from build123d import *

# Parameters (mm, degrees)
PAD_DEPTH                  = 2
PAD001_DEPTH               = 33
POCKET_DEPTH               = 133.8763
POCKET001_DEPTH            = 155.7439
PAD_MIRRORED_2_DEPTH       = 2
PAD001_MIRRORED_2_DEPTH    = 33
POCKET_MIRRORED_2_DEPTH    = 133.8763
POCKET001_MIRRORED_2_DEPTH = 155.7439


with BuildPart() as part:
    # Sketch → Pad (new body)
    with BuildSketch(Plane.XY):
        with BuildLine():
            ThreePointArc((5, 0), (3.535534, 3.535534), (0, 5))
            Line((0, 5), (0, 20))
            Line((0, 20), (39.191836, 20))
            ThreePointArc((41.867601, 13.531593), (40.658555, 16.819092), (39.191836, 20))
            Line((41.867601, 13.531593), (41.867601, 0))
            Line((41.867601, 0), (5, 0))
        make_face()
    pad = extrude(amount=PAD_DEPTH)

    # Sketch001 → Pad001 (join)
    with BuildSketch(Plane.XY):
        with BuildLine():
            ThreePointArc((41.867601, 13.531593), (40.658555, 16.819092), (39.191836, 20))
            Line((0, 20), (39.191836, 20))
            Line((0, 17.6), (0, 20))
            Line((37.030258, 17.6), (0, 17.6))
            ThreePointArc((39.467601, 11.104436), (38.386569, 14.403865), (37.030258, 17.6))
            Line((39.467601, 11.104436), (39.467601, 0))
            Line((39.467601, 0), (41.867601, 0))
            Line((41.867601, 0), (41.867601, 13.531593))
        make_face()
    pad001 = extrude(amount=PAD001_DEPTH)

    # Sketch002 → Pocket (cut, through all)
    with BuildSketch(Plane.XZ):
        Polygon((0, 10), (33.030258, 10), (33.030258, 19), (37.030258, 23), (37.030258, 33), (0, 33), align=None)
    pocket = extrude(amount=-POCKET_DEPTH, mode=Mode.SUBTRACT)

    # Sketch003 → Pocket001 (cut, through all)
    with BuildSketch(Plane.YZ):
        with BuildLine():
            Line((0, 15.000035), (0, 33))
            Line((0, 33), (13, 33))
            Line((13, 28), (13, 33))
            ThreePointArc((0, 15.000035), (9.192376, 18.807634), (13, 28))
        make_face()
    pocket001 = extrude(amount=POCKET001_DEPTH, mode=Mode.SUBTRACT)

    # Sketch Mirrored 2 → Pad Mirrored 2 (add)
    with BuildSketch(Plane(origin=(0, 0, 0), x_dir=(-1, 0, 0), z_dir=(0, 0, -1))):
        with BuildLine():
            ThreePointArc((5, 0), (3.535534, 3.535534), (0, 5))
            Line((0, 5), (0, 20))
            Line((0, 20), (39.191836, 20))
            ThreePointArc((41.867601, 13.531593), (40.658555, 16.819092), (39.191836, 20))
            Line((41.867601, 13.531593), (41.867601, 0))
            Line((41.867601, 0), (5, 0))
        make_face()
    pad_mirrored_2 = extrude(amount=-PAD_MIRRORED_2_DEPTH)

    # Sketch001 Mirrored 2 → Pad001 Mirrored 2 (add)
    with BuildSketch(Plane(origin=(0, 0, 0), x_dir=(-1, 0, 0), z_dir=(0, 0, -1))):
        with BuildLine():
            ThreePointArc((41.867601, 13.531593), (40.658555, 16.819092), (39.191836, 20))
            Line((0, 20), (39.191836, 20))
            Line((0, 17.6), (0, 20))
            Line((37.030258, 17.6), (0, 17.6))
            ThreePointArc((39.467601, 11.104436), (38.386569, 14.403865), (37.030258, 17.6))
            Line((39.467601, 11.104436), (39.467601, 0))
            Line((39.467601, 0), (41.867601, 0))
            Line((41.867601, 0), (41.867601, 13.531593))
        make_face()
    pad001_mirrored_2 = extrude(amount=-PAD001_MIRRORED_2_DEPTH)

    # Sketch002 Mirrored 2 → Pocket Mirrored 2 (cut, through all)
    with BuildSketch(Plane(origin=(0, 0, 0), x_dir=(-1, 0, 0), z_dir=(0, 1, 0))):
        Polygon((0, 10), (33.030258, 10), (33.030258, 19), (37.030258, 23), (37.030258, 33), (0, 33), align=None)
    pocket_mirrored_2 = extrude(amount=POCKET_MIRRORED_2_DEPTH, mode=Mode.SUBTRACT)

    # Sketch003 Mirrored 2 → Pocket001 Mirrored 2 (cut, through all)
    with BuildSketch(Plane.YZ):
        with BuildLine():
            Line((0, 15.000035), (0, 33))
            Line((0, 33), (13, 33))
            Line((13, 28), (13, 33))
            ThreePointArc((0, 15.000035), (9.192376, 18.807634), (13, 28))
        make_face()
    pocket001_mirrored_2 = extrude(amount=-POCKET001_MIRRORED_2_DEPTH, mode=Mode.SUBTRACT)

    # Mirrored001: Pad, Pad001, Pocket, Pocket001, Pad Mirrored 2, Pad001 Mirrored 2, Pocket Mirrored 2, Pocket001 Mirrored 2 across Sketch H_Axis
    add(pad.mirror(Plane.ZX))
    add(pad001.mirror(Plane.ZX))
    add(pocket.mirror(Plane.ZX), mode=Mode.SUBTRACT)
    add(pocket001.mirror(Plane.ZX), mode=Mode.SUBTRACT)
    add(pad_mirrored_2.mirror(Plane.ZX))
    add(pad001_mirrored_2.mirror(Plane.ZX))
    add(pocket_mirrored_2.mirror(Plane.ZX), mode=Mode.SUBTRACT)
    add(pocket001_mirrored_2.mirror(Plane.ZX), mode=Mode.SUBTRACT)


solid = part.part
The model under review builds one solid part; all positions refer to its coordinate system, in mm. A direction names the side the tool comes from. Coordinates: 2 decimals unless noted, no trailing zeros. Loops run counter-clockwise (first coordinate to the right, second up) from the corner with the lowest first, then second, coordinate; pieces in that order, holes last.
(1) Consider section A-A, the plane z = 7. Give the boundary of the cut face in (x, y), plus the area to 3 significant figures.
Determined:
outline: (-41.87, -13.53) arc R44 ccw to (-39.19, -20) - (39.19, -20) arc R44 ccw to (41.87, -13.53) - (41.87, 13.53) arc R44 ccw to (39.19, 20) - (-39.19, 20) arc R44 ccw to (-41.87, 13.53) - close; hole (-39.47, -11.1) arc R41 ccw to (-37.03, -17.6) - (37.03, -17.6) arc R41 ccw to (39.47, -11.1) - (39.47, 11.1) arc R41 ccw to (37.03, 17.6) - (-37.03, 17.6) arc R41 ccw to (-39.47, 11.1) - close
area: 568 mm2
(2) Draft analysis for pull direction Y (two halves, no side actions). For faces 6 (the flat face through (40, 13, 30)), 7 (the cylindrical face through (40.68, -16.77, 16.27)), 8 (the flat face through (39, -17, 33)), state which applies: +Y half, -Y half, draft (parallel to the pull), parting line (faces both ways), or undercut.
Determined:
face 6: undercut
face 7: -Y half
face 8: draft
(3) Wall thickness on L1, parallel to Y at x = 21, z = 3; L2, parallel to X at y = 8, z = 7; L3, parallel to X at y = -13, z = 10.5: over which ranges is each line inside the solid? List them lowest first.
Determined:
L1: y = -20 to -17.6, 17.6 to 20
L2: x = -41.87 to -39.47, 39.47 to 41.87
L3: x = -41.87 to -38.88, 38.88 to 41.87
(4) Insertion check: P1, Ø1.9, axis at y = -19, z = 15, coming from the -X side; P2, Ø0.7, axis at y = -18.5, z = 16, coming from the +X side; P3, Ø2.5, axis at x = 41, z = 30.5, coming from the -Y side. Each pin has a flat end and moves straight along its axis. Give the tip position at first contact, or say it passes through.
Determined:
P1: stops at x = -40.13
P2: stops at x = 40.08
P3: stops at y = -18.87
(5) Consider section D-D, the plane x = 13. Give the boundary of the cut face in (y, z), plus the area to 3 significant figures.
Determined:
outline: (-20, 0) - (20, 0) - (20, 10) - (17.6, 10) - (17.6, 2) - (-17.6, 2) - (-17.6, 10) - (-20, 10) - close
area: 118 mm2
(6) Consider section B-B, the plane y = -3.5. Give the boundary of the cut face in (x, z).
Determined:
outline: (-41.87, 0) - (-3.57, 0) - (-3.57, 2) - (-39.47, 2) - (-39.47, 15.48) - (-41.87, 15.48) - close; (3.57, 0) - (41.87, 0) - (41.87, 15.48) - (39.47, 15.48) - (39.47, 2) - (3.57, 2) - close
(7) Tool access review of faces 1 (the flat face through (0, -19, 10)), 2 (the flat face through (-39.468, 0, 9)), 3 (the flat face through (-39, -17, 33)), 4 (the flat face through (-1, -9, 0)), 5 (the flat face through (-40, 13, 30)): name each direction out of +Z, -Z, +X, -X, +Y, -Y from which nothing blocks a thin tool from reaching the whole face with its end or side.
Determined:
face 1: +Z, +Y, -Y
face 2: +Z
face 3: +Z, +X, -X, +Y, -Y
face 4: -Z, +X, -X, +Y, -Y
face 5: +Z, +X, -X
(8) Consider section C-C, the plane z = 30. Give the boundary of the cut face in (x, y), plus the area to 3 significant figures.
Determined:
outline: (-41.87, -13.53) arc R44 ccw to (-39.19, -20) - (-37.03, -20) - (-37.03, -17.6) arc R41 cw to (-38.88, -13) - (-41.87, -13) - close; (-41.87, 13) - (-38.88, 13) arc R41 cw to (-37.03, 17.6) - (-37.03, 20) - (-39.19, 20) arc R44 ccw to (-41.87, 13.53) - close; (37.03, -20) - (39.19, -20) arc R44 ccw to (41.87, -13.53) - (41.87, -13) - (38.88, -13) arc R41 cw to (37.03, -17.6) - close; (37.03, 17.6) arc R41 cw to (38.88, 13) - (41.87, 13) - (41.87, 13.53) arc R44 ccw to (39.19, 20) - (37.03, 20) - close
area: 85.4 mm2
